Design review of the part built by this model. Coordinates are the model's own, in mm. A direction names the side the tool comes from. Coordinates: 2 decimals unless noted, no trailing zeros. Loops run counter-clockwise (first coordinate to the right, second up) from the corner with the lowest first, then second, coordinate; pieces in that order, holes last. Notation, with made-up numbers: (55, 31.5) -> (73, 31.5) arc R17 cw to (73, 46.5) -> close; hole circle Ø6 at (70, 77). An arc over 180 degrees is marked (long way). Answer in a Markdown table with one row per item.
```python
from build123d import *

# Parameters (mm, degrees)
F0_W      = 50
F0_H      = 50
F1_DEPTH  = 50
F2_W      = 10
F2_H      = 40
F3_DEPTH  = 40
F6_R      = 10
F7_DEPTH  = 6
F9_DEPTH  = 20
F14_DEPTH = 10
F15_SIZE  = 10


with BuildPart() as f1:
    # F0 (on Top) → F1 (new body)
    with BuildSketch(Plane.XY):
        with Locations((25, 25)):
            Rectangle(F0_W, F0_H)
    extrude(amount=F1_DEPTH)

    # F2 (on face) → F3 (cut)
    with BuildSketch(Plane.XY.offset(50)):
        with Locations((39, 20)):
            Rectangle(F2_W, F2_H)
    extrude(amount=-F3_DEPTH, mode=Mode.SUBTRACT)

    # F6
    f6_edges = [f1.edges().sort_by_distance(p)[0] for p in [
        (39, 40, 10),
    ]]
    fillet(f6_edges, radius=F6_R)

    # F5 (on face) → F7 (cut)
    with BuildSketch(Plane.YZ.offset(50)):
        Polygon((0, 50), (0, 30), (20, 50), align=None)
    extrude(amount=-F7_DEPTH, mode=Mode.SUBTRACT)

    # F8 (on face) → F9 (cut)
    with BuildSketch(Plane(origin=(0, 0, 0), x_dir=(1, 0, 0), z_dir=(0, 0, -1))):
        with BuildLine():
            ThreePointArc((0, -25), (17.6776695297, -17.6776695297), (25, 0))
            Line((25, 0), (0, 0))
            Line((0, 0), (0, -25))
        make_face()
    extrude(amount=-F9_DEPTH, mode=Mode.SUBTRACT)

    # F9_face (on face) → F11 section 0
    with BuildSketch(Plane(origin=(10.6103295395, 10.6103295395, 20), x_dir=(1, 0, 0), z_dir=(0, 0, -1)), mode=Mode.PRIVATE) as f11_s0:
        with BuildLine():
            ThreePointArc((-10.6103295395, -14.3896704605), (7.0673399902, -7.0673399902), (14.3896704605, 10.6103295395))
            Line((14.3896704605, 10.6103295395), (-10.6103295395, 10.6103295395))
            Line((-10.6103295395, 10.6103295395), (-10.6103295395, -14.3896704605))
        make_face()
    loft([f11_s0.sketch, Vertex(0, 0, 50.0027686357)], mode=Mode.SUBTRACT)

    # F13 (on face) → F14 (cut)
    with BuildSketch(Plane.XY.offset(50)):
        with BuildLine():
            ThreePointArc((0, 15), (10.6066017178, 10.6066017178), (15, 0))
            Line((15, 0), (25, 0))
            Line((25, 0), (25, 25))
            Line((25, 25), (0, 25))
            Line((0, 25), (0, 15))
        make_face()
    extrude(amount=-F14_DEPTH, mode=Mode.SUBTRACT)

    # F15
    f15_edges = [f1.edges().sort_by_distance(p)[0] for p in [
        (25, 25, 45),
    ]]
    chamfer(f15_edges, length=F15_SIZE)


solid = f1.part
```
(1) Take a section at B-B on x = 39. Give the boundary of the cut face in (y, z).
Evaluation:
| item | result |
|---|---|
| outline | (0, 0) -> (50, 0) -> (50, 50) -> (40, 50) -> (40, 20) arc R10 cw to (30, 10) -> (0, 10) -> close |
(2) Take a section at A-A on y = 27. Give the boundary of the cut face in (x, z).
Evaluation:
| item | result |
|---|---|
| outline | (0, 0) -> (50, 0) -> (50, 50) -> (44, 50) -> (44, 10) -> (34, 10) -> (34, 50) -> (0, 50) -> close |
(3) Take a section at D-D on z = 19. Give the boundary of the cut face in (x, y).
Evaluation:
| item | result |
|---|---|
| outline | (0, 25) arc R25 cw to (25, 0) -> (34, 0) -> (34, 39.95) -> (44, 39.95) -> (44, 0) -> (50, 0) -> (50, 50) -> (0, 50) -> close |
(4) Draft analysis for pull direction X (two halves, no side actions). For faces 5 (the cylindrical face through (17.482, 17.871, 9.86)), 6 (the flat face through (47, 10, 40)), 7 (the flat face through (15, 15, 40)), state which applies: pulls with the +X half, pulls with the -X half, needs draft (parallel to the pull), parting line crosses it, or undercut.
Evaluation:
| item | result |
|---|---|
| face 5 | pulls with the -X half |
| face 6 | needs draft |
| face 7 | undercut |
(5) Take a section at C-C on z = 11. Give the boundary of the cut face in (x, y).
Evaluation:
| item | result |
|---|---|
| outline | (0, 25) arc R25 cw to (25, 0) -> (34, 0) -> (34, 34.36) -> (44, 34.36) -> (44, 0) -> (50, 0) -> (50, 50) -> (0, 50) -> close |
(6) For pin 1 (3 mm diameter, centred on x = 19.5, z = 20, fed in from -Y); pin 2 (3 mm diameter, centred on x = 38, z = 33.5, fed in from -Y), all flat-tipped, find the tip position at first contact; note any pin that passes through.
Evaluation:
| item | result |
|---|---|
| pin 1 | stops at y = 12.6 |
| pin 2 | stops at y = 40 |
(7) Tool access review of faces 1 (the cylindrical face through (10.49, 10.72, 45.07)), 2 (the flat face through (44, 20, 30)), 3 (the flat face through (20, 20, 45)), 4 (the flat face through (8, 25, 45)): name each direction out of +Z, -Z, +X, -X, +Y, -Y from which nothing blocks a thin tool from reaching the whole face with its end or side.
Evaluation:
| item | result |
|---|---|
| face 1 | +Z |
| face 2 | +Z, -Y |
| face 3 | +Z, -X, -Y |
| face 4 | +Z, -X |
(8) To check wall thickness, follow probe 1 along X at (y, z) = (16.5, 31.5); probe 2 along Z at (x, y) = (41, 11); probe 3 along X at (y, z) = (10, 35). State the ranges of each line that lie inside material, in increasing order.
Evaluation:
| item | result |
|---|---|
| probe 1 | x = 0 to 34, 44 to 50 |
| probe 2 | z = 0 to 10 |
| probe 3 | x = 7.5 to 34, 44 to 50 |
